Work out the finished part from the listing and answer in its coordinate system (mm). A direction names the side the tool comes from. Give positions to 0.01 mm unless a question says otherwise; leave off trailing zeros. Order: outer loops, then holes, each group sorted by start corner. A loop starts at its lowest first (then second) coordinate and runs counter-clockwise, first axis right, second up. Notation, with made-up numbers: M 66.25,-34.75 L 113.25,-34.75 A27 ccw 113.25,3.25 Z; hole C 74.5,-26.5 d8. An arc over 180 degrees is marked long. One line per item, written item: value.
from build123d import *

# Parameters (mm, degrees)
SKETCH1_W           = 30.5
SKETCH1_H           = 39.5
SKETCH1_W_2         = 26.5
SKETCH1_H_2         = 35.5
BOSS_EXTRUDE1_DEPTH = 22
SKETCH3_W           = 26.5
SKETCH3_H           = 35.5
SKETCH3_W_2         = 22.3
SKETCH3_H_2         = 31.3
BOSS_EXTRUDE3_DEPTH = 11.75
BOSS_EXTRUDE4_START = -22
SKETCH4_R           = 1.55
BOSS_EXTRUDE4_DEPTH = 4
CUT_EXTRUDE1_DEPTH  = 2
CHAMFER2_SIZE       = 3
CUT_EXTRUDE2_DEPTH  = 71.029433394
CUT_EXTRUDE3_START  = -2
CUT_EXTRUDE3_DEPTH  = 2
CHAMFER3_SIZE       = 2


with BuildPart() as part:
    # Sketch1 → Boss-Extrude1 (new body)
    with BuildSketch(Plane(origin=(0, 0, 0), x_dir=(1, 0, 0), z_dir=(0, 1, 0))):
        Rectangle(SKETCH1_W, SKETCH1_H)
        Rectangle(SKETCH1_W_2, SKETCH1_H_2, mode=Mode.SUBTRACT)
    extrude(amount=BOSS_EXTRUDE1_DEPTH)

    # Sketch3 → Boss-Extrude3 (add)
    with BuildSketch(Plane.XZ):
        Rectangle(SKETCH3_W, SKETCH3_H)
        Rectangle(SKETCH3_W_2, SKETCH3_H_2, mode=Mode.SUBTRACT)
    extrude(amount=-BOSS_EXTRUDE3_DEPTH)

    # Sketch4 → Boss-Extrude4 (add)
    # profile 1 of 2: a face of its own
    with BuildSketch(Plane(origin=(0, 22, 0), x_dir=(1, 0, 0), z_dir=(0, 1, 0)).offset(BOSS_EXTRUDE4_START)):
        with BuildLine():
            Line((-33.257041555, -32.927114317), (-10.433610061, -19.75))
            Line((-10.433610061, -19.75), (-15.25, -19.75))
            Line((-15.25, -19.75), (-15.25, -12.138439182))
            Line((-15.25, -12.138439182), (-37.757041555, -25.132885683))
            ThreePointArc((-37.757041555, -25.132885683), (-39.404155872, -31.28), (-33.257041555, -32.927114317))
        make_face()
        with Locations(Location((-35.507041555, -29.03, 0), (0, 0, 270))):
            Circle(SKETCH4_R, mode=Mode.SUBTRACT)
    # profile 2 of 2: a face of its own
    with BuildSketch(Plane(origin=(0, 22, 0), x_dir=(1, 0, 0), z_dir=(0, 1, 0)).offset(BOSS_EXTRUDE4_START)):
        with BuildLine():
            Line((-4.5, 19.75), (4.5, 19.75))
            Line((4.5, 19.75), (4.5, 32.47))
            ThreePointArc((4.5, 32.47), (0, 36.97), (-4.5, 32.47))
            Line((-4.5, 32.47), (-4.5, 19.75))
        make_face()
        with Locations(Location((0, 32.47, 0), (0, 0, 270))):
            Circle(SKETCH4_R, mode=Mode.SUBTRACT)
    boss_extrude4 = extrude(amount=BOSS_EXTRUDE4_DEPTH)

    # Sketch6 → Cut-Extrude1 (cut)
    with BuildSketch(Plane(origin=(0, 4, 0), x_dir=(1, 0, 0), z_dir=(0, 1, 0))):
        Polygon((-2.85, 34.115448267), (-2.85, 30.824551733), (0, 29.179103466), (2.85, 30.824551733), (2.85, 34.115448267), (0, 35.760896534), align=None)
        Polygon((-35.507041555, -32.320896534), (-32.657041555, -30.675448267), (-32.657041555, -27.384551733), (-35.507041555, -25.739103466), (-38.357041555, -27.384551733), (-38.357041555, -30.675448267), align=None)
    cut_extrude1 = extrude(amount=-CUT_EXTRUDE1_DEPTH, mode=Mode.SUBTRACT)

    # Mirror1: Boss-Extrude4, Cut-Extrude1 across plane
    add(boss_extrude4.mirror(Plane(origin=(0, 0, 0), x_dir=(0, 0, 1), z_dir=(1, 0, 0))))
    add(cut_extrude1.mirror(Plane(origin=(0, 0, 0), x_dir=(0, 0, 1), z_dir=(1, 0, 0))), mode=Mode.SUBTRACT)

    # Chamfer2
    # the kernel refuses this chamfer: 3 mm, written as the material it adds along each edge
    with BuildSketch(Plane(origin=(15.25, 4, 19.75), x_dir=(0, 1, 0), z_dir=(0, 0, -1))) as chamfer2_piece_1_section:
        Polygon((CHAMFER2_SIZE, 0), (0, CHAMFER2_SIZE), (0, 0), align=None)
    chamfer2_piece_1 = extrude(amount=15.326609781, mode=Mode.PRIVATE)
    chamfer2_piece_1 = split(chamfer2_piece_1, bisect_by=Plane(origin=(18.545902515, 4, 14.041329387), z_dir=(-0.4999999999999982, 0, 0.8660254037844397)), keep=Keep.TOP, mode=Mode.PRIVATE)
    add(chamfer2_piece_1)
    with BuildSketch(Plane(origin=(2.718561097, 4, 19.75), x_dir=(0, 1, 0), z_dir=(1, 0, 0))) as chamfer2_piece_2_section:
        Polygon((CHAMFER2_SIZE, 0), (0, CHAMFER2_SIZE), (0, 0), align=None)
    chamfer2_piece_2 = extrude(amount=12.531438903, mode=Mode.PRIVATE)
    chamfer2_piece_2 = split(chamfer2_piece_2, bisect_by=Plane(origin=(4.647323338, 4, 16.409285803), z_dir=(0.4999999999999978, 0, -0.8660254037844399)), keep=Keep.TOP, mode=Mode.PRIVATE)
    add(chamfer2_piece_2)
    with BuildSketch(Plane(origin=(-4.5, 4, -19.75), x_dir=(0, 1, 0), z_dir=(1, 0, 0))) as chamfer2_piece_3:
        Polygon((CHAMFER2_SIZE, 0), (0, -CHAMFER2_SIZE), (0, 0), align=None)
    extrude(amount=9)
    with BuildSketch(Plane(origin=(-15.25, 4, 19.75), x_dir=(0, 1, 0), z_dir=(0, 0, -1))) as chamfer2_piece_4_section:
        Polygon((CHAMFER2_SIZE, 0), (0, -CHAMFER2_SIZE), (0, 0), align=None)
    chamfer2_piece_4 = extrude(amount=15.326609781, mode=Mode.PRIVATE)
    chamfer2_piece_4 = split(chamfer2_piece_4, bisect_by=Plane(origin=(-18.545902515, 4, 14.041329387), z_dir=(0.4999999999999982, 0, 0.8660254037844397)), keep=Keep.TOP, mode=Mode.PRIVATE)
    add(chamfer2_piece_4)
    with BuildSketch(Plane(origin=(-2.718561097, 4, 19.75), x_dir=(0, 1, 0), z_dir=(-1, 0, 0))) as chamfer2_piece_5_section:
        Polygon((CHAMFER2_SIZE, 0), (0, -CHAMFER2_SIZE), (0, 0), align=None)
    chamfer2_piece_5 = extrude(amount=12.531438903, mode=Mode.PRIVATE)
    chamfer2_piece_5 = split(chamfer2_piece_5, bisect_by=Plane(origin=(-4.647323338, 4, 16.409285803), z_dir=(-0.4999999999999978, 0, -0.8660254037844399)), keep=Keep.TOP, mode=Mode.PRIVATE)
    add(chamfer2_piece_5)
    with BuildSketch(Plane(origin=(15.25, 4, 27.465048964), x_dir=(0, 1, 0), z_dir=(0, 0, -1))) as chamfer2_piece_6a_section:
        Polygon((CHAMFER2_SIZE, 0), (0, CHAMFER2_SIZE), (0, 0), align=None)
    chamfer2_piece_6a = extrude(amount=23.041658745, mode=Mode.PRIVATE)
    chamfer2_piece_6a = split(chamfer2_piece_6a, bisect_by=Plane(origin=(15.25, 4, 19.75), z_dir=(0, 0, 1)), keep=Keep.TOP, mode=Mode.PRIVATE)
    chamfer2_piece_6a = split(chamfer2_piece_6a, bisect_by=Plane(origin=(17.386616712, 4, 23.764320262), z_dir=(0.4999999999999978, 0, -0.8660254037844399)), keep=Keep.TOP, mode=Mode.PRIVATE)
    with BuildSketch(Plane(origin=(2.718561097, 4, 19.75), x_dir=(0, 1, 0), z_dir=(1, 0, 0))) as chamfer2_piece_6b_section:
        Polygon((CHAMFER2_SIZE, 0), (0, CHAMFER2_SIZE), (0, 0), align=None)
    chamfer2_piece_6b = extrude(amount=20.246487867, mode=Mode.PRIVATE)
    chamfer2_piece_6b = split(chamfer2_piece_6b, bisect_by=Plane(origin=(15.25, 4, 19.75), z_dir=(1, 0, 0)), keep=Keep.TOP, mode=Mode.PRIVATE)
    chamfer2_piece_6b = split(chamfer2_piece_6b, bisect_by=Plane(origin=(4.647323338, 4, 16.409285803), z_dir=(0.4999999999999978, 0, -0.8660254037844399)), keep=Keep.TOP, mode=Mode.PRIVATE)
    chamfer2_piece_6 = chamfer2_piece_6a & chamfer2_piece_6b
    add(chamfer2_piece_6)
    with BuildSketch(Plane(origin=(-15.25, 4, 27.465048964), x_dir=(0, 1, 0), z_dir=(0, 0, -1))) as chamfer2_piece_7a_section:
        Polygon((CHAMFER2_SIZE, 0), (0, -CHAMFER2_SIZE), (0, 0), align=None)
    chamfer2_piece_7a = extrude(amount=23.041658745, mode=Mode.PRIVATE)
    chamfer2_piece_7a = split(chamfer2_piece_7a, bisect_by=Plane(origin=(-17.386616712, 4, 23.764320262), z_dir=(-0.4999999999999978, 0, -0.8660254037844399)), keep=Keep.TOP, mode=Mode.PRIVATE)
    chamfer2_piece_7a = split(chamfer2_piece_7a, bisect_by=Plane(origin=(-15.25, 4, 19.75), z_dir=(0, 0, 1)), keep=Keep.TOP, mode=Mode.PRIVATE)
    with BuildSketch(Plane(origin=(-2.718561097, 4, 19.75), x_dir=(0, 1, 0), z_dir=(-1, 0, 0))) as chamfer2_piece_7b_section:
        Polygon((CHAMFER2_SIZE, 0), (0, -CHAMFER2_SIZE), (0, 0), align=None)
    chamfer2_piece_7b = extrude(amount=20.246487867, mode=Mode.PRIVATE)
    chamfer2_piece_7b = split(chamfer2_piece_7b, bisect_by=Plane(origin=(-15.25, 4, 19.75), z_dir=(-1, 0, 0)), keep=Keep.TOP, mode=Mode.PRIVATE)
    chamfer2_piece_7b = split(chamfer2_piece_7b, bisect_by=Plane(origin=(-4.647323338, 4, 16.409285803), z_dir=(-0.4999999999999978, 0, -0.8660254037844399)), keep=Keep.TOP, mode=Mode.PRIVATE)
    chamfer2_piece_7 = chamfer2_piece_7a & chamfer2_piece_7b
    add(chamfer2_piece_7)

    # Sketch7 → Cut-Extrude2 (cut, through all)
    with BuildSketch(Plane(origin=(15.25, 0, 0), x_dir=(0, 0, -1), z_dir=(1, 0, 0))):
        with BuildLine():
            Line((5.55, 0), (-2.05, 0))
            Line((-2.05, 0), (-2.05, 5))
            ThreePointArc((-2.05, 5), (-1.757106781, 5.707106781), (-1.05, 6))
            Line((-1.05, 6), (4.55, 6))
            ThreePointArc((4.55, 6), (5.257106781, 5.707106781), (5.55, 5))
            Line((5.55, 5), (5.55, 0))
        make_face()
    extrude(amount=-CUT_EXTRUDE2_DEPTH, mode=Mode.SUBTRACT)

    # Sketch8 → Cut-Extrude3 (cut)
    with BuildSketch(Plane(origin=(0, 4, 0), x_dir=(1, 0, 0), z_dir=(0, 1, 0)).offset(CUT_EXTRUDE3_START)):
        with BuildLine():
            Line((-34.474028853, -23.237437416), (-29.974028853, -31.03166605))
            Line((-29.974028853, -31.03166605), (-33.257041555, -32.927114317))
            ThreePointArc((-33.257041555, -32.927114317), (-39.404155872, -31.28), (-37.757041555, -25.132885683))
            Line((-37.757041555, -25.132885683), (-34.474028853, -23.237437416))
        make_face()
        with BuildLine():
            Line((4.5, 28.679103466), (4.5, 32.47))
            ThreePointArc((4.5, 32.47), (0, 36.97), (-4.5, 32.47))
            Line((-4.5, 32.47), (-4.5, 28.679103466))
            Line((-4.5, 28.679103466), (4.5, 28.679103466))
        make_face()
        with BuildLine():
            Line((33.257041555, -32.927114317), (29.974028853, -31.03166605))
            Line((29.974028853, -31.03166605), (34.474028853, -23.237437416))
            Line((34.474028853, -23.237437416), (37.757041555, -25.132885683))
            ThreePointArc((37.757041555, -25.132885683), (39.404155872, -31.28), (33.257041555, -32.927114317))
        make_face()
    extrude(amount=CUT_EXTRUDE3_DEPTH, mode=Mode.SUBTRACT)

    # Chamfer3
    chamfer3_edges = [part.edges().sort_by_distance(p)[0] for p in [
        (-34.474028853, 3, 23.237437416),
        (-29.974028853, 3, 31.03166605),
        (4.5, 3, -28.679103466),
        (-4.5, 3, -28.679103466),
        (29.974028853, 3, 31.03166605),
        (34.474028853, 3, 23.237437416),
    ]]
    chamfer(chamfer3_edges, length=CHAMFER3_SIZE)


solid = part.part
(1) Section C-C, the plane y = 8.25 is taken. Give the vertices of the cut face in (x, z).
Findings:
outline: M -15.25,-19.75 L 15.25,-19.75 L 15.25,19.75 L -15.25,19.75 Z; hole M -11.15,-15.65 L 11.15,-15.65 L 11.15,15.65 L -11.15,15.65 Z
(2) Section D-D, the plane x = -23.5 is taken. Give the vertices of the cut face in (y, z), then the cut area to 3 significant figures.
Findings:
outline: M 0,16.9 L 4,16.9 L 4,27.29 L 0,27.29 Z
area: 41.6 mm^2
(3) Find the intervals of material crossed by probe 1 along Z at (x, y) = (0, 1.65); probe 2 along Z at (x, y) = (-6, 19.5); probe 3 along X at (y, z) = (8.5, 10), in increasing order. Write a range as from..to.
Findings:
probe 1: z = -36.97..-34.02, -30.92..-15.65, 15.65..19.75
probe 2: z = -19.75..-17.75, 17.75..19.75
probe 3: x = -15.25..-11.15, 11.15..15.25
(4) Section A-A, the plane x = 7.5 is taken. Give the vertices of the cut face in (y, z).
Findings:
outline: M 0,-19.75 L 22,-19.75 L 22,-17.75 L 11.75,-17.75 L 11.75,-15.65 L 0,-15.65 Z; M 0,15.65 L 11.75,15.65 L 11.75,17.75 L 22,17.75 L 22,19.75 L 0,19.75 Z
(5) Determine the mould class of faces 1 (the cylindrical face through (36.45, 0.99, 27.8)), 2 (the flat face through (16.73, 5.52, 17.52)), 3 (the flat face through (-16.73, 5.52, 17.52)), 4 (the flat face through (-13, 2, 2.05)) for opening direction X: pulls with the +X half, pulls with the -X half, needs draft (parallel to the pull), parting line crosses it, or undercut.
Findings:
face 1: undercut
face 2: pulls with the +X half
face 3: pulls with the -X half
face 4: needs draft
(6) Section B-B, the plane y = 15.25 is taken. Give the vertices of the cut face in (x, z).
Findings:
outline: M -15.25,-19.75 L 15.25,-19.75 L 15.25,19.75 L -15.25,19.75 Z; hole M -13.25,-17.75 L 13.25,-17.75 L 13.25,17.75 L -13.25,17.75 Z
(7) Given P1, Ø4.5, axis at x = 1.5, z = -30.5, coming from the +Y side; P2, Ø3, axis at x = -1.5, y = 18.5, coming from the -Z side; P3, Ø4.5, axis at x = 0.5, z = -24.5, coming from the +Y side; P4, Ø3, axis at x = -18.5, z = -12.5, coming from the +Y side, each flat-ended and moving along its own axis, determine where each tip first touches the part or whether it passes through.
Findings:
P1: stops at y = 4
P2: stops at z = -19.75
P3: stops at y = 4.5
P4: passes through
(8) Which of the six approach directions +Z, -Z, +X, -X, +Y, -Y give full straight-line access (tool end or side, diameter ignored) to faces 5 (the flat face through (-13, 3, -5.55)), 6 (the flat face through (0, 3, -28.679)), 7 (the flat face through (32.21, 2.99, 27.16))?
Findings:
face 5: +X, -X, -Y
face 6: -Z, +X, -X, +Y
face 7: +Z, +X, +Y
